Autodesk Inventor part; units mm, degrees
ref_plane "YZ Plane" through (0, 0, 0) normal (1, 0, 0) x (0, 1, 0)
ref_plane "XZ Plane" through (0, 0, 0) normal (0, 1, 0) x (-1, 0, 0)
ref_plane "XY Plane" through (0, 0, 0) normal (0, 0, 1) x (1, 0, 0)
sketch "Sketch1" plane through (0, 0, 0) normal (0, 0, 1) x (1, 0, 0)
  line L0 (0, 0) -> (4, 0)
  line L1 (4, 0) -> (4, -20)
  line L2 (4, -20) -> (0, -20)
  line L3 (0, -20) -> (0, 0)
  circle A0 centre (4, -4) radius 2.5
  circle A1 centre (4, -16) radius 2.5
  line L4 (1.5, -4) -> (1.5, -7)
  line L5 (1.5, -7) -> (1.5, -1)
  line L6 (4, -7) -> (1.5, -7)
  line L7 (1.5, -1) -> (4, -1)
  point P0 (4, -18.5)
  point P1 (4, -13.5)
  dimension "d2" = 5
  dimension "d0" = 20
  dimension "d1" = 4
  dimension "d3" = 5
  dimension "d4" = 4
  dimension "d5" = 4
  dimension "d6" = 3
  dimension "d7" = 3
extrude "Extrusion1" add sketch "Sketch1" along normal blind 5 contours L0 L1 L7 L5 L4 L6 A1 L2 L3
sketch "Sketch3" plane through (0, -20, 0) normal (-1, 0, 0) x (0, 0, 1)
  circle A0 centre (2.5, 10) radius 1.35
  line L0 (0, 0) -> (5, 0)
  line L1 (0, 20) -> (0, 0)
  dimension "d10" = 10
  dimension "d11" = 2.5
  dimension "d12" = 20
  dimension "d13" = 2.7
extrude "Extrusion2" cut sketch "Sketch3" against normal blind 20
sketch "Sketch4" plane through (0, -20, 0) normal (-1, 0, 0) x (0, 0, 1)
  circle A0 centre (2.5, 10) radius 1.35
  circle A1 centre (2.5, 10) radius 2.45
  point P0 (0, 20)
  dimension "d16" = 4.9
extrude "Extrusion3" cut sketch "Sketch4" against normal blind 2.5 contours A0 | A1
equation "\"d1\" = d4"
properties part number "POMSliderAxis" material "Acetal Resin, White"
The listing builds one solid part. Answer for the finished solid, in the listing's coordinates (mm). A direction names the side the tool comes from. Round coordinates to 2 decimals unless told otherwise and drop trailing zeros. Loops run counter-clockwise (first coordinate to the right, second up) from the corner with the lowest first, then second, coordinate; pieces in that order, holes last. Notation, with made-up numbers: (-37.5, 23.5) - (19.5, 23.5) arc R13 ccw to (19.5, 35.5) - close; hole circle Ø1 at (-9.75, 55). An arc over 180 degrees is marked (long way). Return JSON: item names as keys, results as strings. Group by question number.
1. Each of these flat-tipped pins is pushed along its axis until it touches: P1, Ø2.5, axis at y = -2.5, z = 1.5, coming from the +X side; P2, Ø3, axis at y = -10, z = 2.5, coming from the -X side. Where does it stop, or does it pass through?
2. Consider probe 1 along Y at (x, z) = (3.4, 4.2); probe 2 along Y at (x, z) = (2.05, 3.15); probe 3 along Y at (x, z) = (2.65, 3.7). Determine where each line is inside the solid, lowest interval first.
3. The part is cut by section B-B on x = 2.9. Determine the outline of the cut face in (y, z) (3 decimals), then the cut area to 3 significant figures.
4. The part is cut by section A-A on z = 2.5. Determine the outline of the cut face in (x, y), then the cut area to 3 significant figures.
5. Which of the six approach directions +Z, -Z, +X, -X, +Y, -Y give full straight-line access (tool end or side, diameter ignored) to faces 1 (the cylindrical face through (1.2, -12.4, 2)), 2 (the flat face through (1.5, -4, 2)), 3 (the flat face through (2, -20, 2))?
6. The part is cut by section C-C on x = 1.3. Determine the outline of the cut face in (y, z).
7. The part is cut by section D-D on z = 0.7. Determine the outline of the cut face in (x, y).
8. The mould has two halves that part along Z. Classify faces 4 (the flat face through (3, -10, 5)), 5 (the flat face through (4, -19, 2)), 6 (the flat face through (2.5, -11, 4)): pulls with the +Z half, pulls with the -Z half, needs draft (parallel to the pull), parting line crosses it, or undercut.
Resolved:
{
 "1": {"P1": "stops at x = 1.5", "P2": "stops at x = 2.5"},
 "2": {"probe 1": "y = -20 to -18.43, -13.57 to -7, -1 to 0", "probe 2": "y = -20 to -17.56, -14.44 to -12.36, -7.64 to -7, -1 to 0", "probe 3": "y = -20 to -18.1, -13.9 to -10.62, -9.38 to -7, -1 to 0"},
 "3": {"outline": "(-20, 0) - (-18.245, 0) - (-18.245, 5) - (-20, 5) - close; (-13.755, 0) - (-7, 0) - (-7, 5) - (-13.755, 5) - close; (-1, 0) - (0, 0) - (0, 5) - (-1, 5) - close; hole circle Ø2.7 at (-10, 2.5)", "area": "41.8 mm²"},
 "4": {"outline": "(0, -20) - (4, -20) - (4, -18.5) arc R2.5 cw to (4, -13.5) - (4, -11.35) - (2.5, -11.35) - (2.5, -12.45) - (0, -12.45) - close; (0, -7.55) - (2.5, -7.55) - (2.5, -8.65) - (4, -8.65) - (4, -7) - (1.5, -7) - (1.5, -1) - (4, -1) - (4, 0) - (0, 0) - close", "area": "38.9 mm²"},
 "5": {"face 1": "-X", "face 2": "+Z, -Z, +X", "face 3": "+Z, -Z, +X, -X, -Y"},
 "6": {"outline": "(-20, 0) - (0, 0) - (0, 5) - (-20, 5) - close; hole circle Ø4.9 at (-10, 2.5)"},
 "7": {"outline": "(0, -20) - (4, -20) - (4, -18.5) arc R2.5 cw to (4, -13.5) - (4, -7) - (1.5, -7) - (1.5, -1) - (4, -1) - (4, 0) - (0, 0) - (0, -8.34) - (2.5, -8.34) - (2.5, -11.66) - (0, -11.66) - close"},
 "8": {"face 4": "pulls with the +Z half", "face 5": "needs draft", "face 6": "undercut"}
}
